Part model, mm, in its own coordinate system. Give positions to 0.01 mm unless a question says otherwise; leave off trailing zeros. Loops run counter-clockwise (first coordinate to the right, second up) from the corner with the lowest first, then second, coordinate; pieces in that order, holes last. Notation, with made-up numbers: M 45,60 L 88,60 A19 cw 88,88 Z; hole C 2,71 d2. An arc over 180 degrees is marked long. Put each result on its own line as item: value. Start each with the question number.
```python
from build123d import *

# Parameters (mm, degrees)
SKETCH1_R                        = 101.6
SKETCH1_R_2                      = 22.225
BOSS_EXTRUDE1_DEPTH              = 12.7
F_1_4_20_TAPPED_HOLE1_AT_2_COUNT = 2
F_1_4_20_TAPPED_HOLE1_AT_2_PITCH = 91.581002397
F_1_4_20_TAPPED_HOLE1_AT_3_COUNT = 2
F_1_4_20_TAPPED_HOLE1_AT_3_PITCH = 71.842048969
F_1_4_20_TAPPED_HOLE1_AT_4_COUNT = 2
F_1_4_20_TAPPED_HOLE1_AT_4_PITCH = 127
F_1_4_20_TAPPED_HOLE1_AT_5_COUNT = 2
F_1_4_20_TAPPED_HOLE1_AT_5_PITCH = 101.6
F_1_4_20_TAPPED_HOLE1_AT_6_COUNT = 2
F_1_4_20_TAPPED_HOLE1_AT_6_PITCH = 91.581002397
F_1_4_20_TAPPED_HOLE1_AT_7_COUNT = 2
F_1_4_20_TAPPED_HOLE1_AT_7_PITCH = 71.842048969
F_1_4_20_TAPPED_HOLE1_AT_8_COUNT = 2
F_1_4_20_TAPPED_HOLE1_AT_8_PITCH = 25.4


with BuildPart() as part:
    # Sketch1 → Boss-Extrude1 (new body)
    with BuildSketch(Plane.XY):
        Circle(SKETCH1_R)
        Circle(SKETCH1_R_2, mode=Mode.SUBTRACT)
    extrude(amount=BOSS_EXTRUDE1_DEPTH)

    # Sketch3 → 1/4-20 Tapped Hole1 (revolve, cut)
    with BuildSketch(Plane(origin=(-50.8, 0, 12.7), x_dir=(0, -1, 0), z_dir=(1, 0, 0))):
        Polygon((0, 0), (0, 12.7), (3.81, 12.7), (2.5527, 11.4427), (2.5527, 1.2573), (3.81, 0), align=None)
    f_1_4_20_tapped_hole1 = revolve(axis=Axis((-50.8, 0, 19.05), (0, 0, -1)), mode=Mode.SUBTRACT)

    # 1/4-20 Tapped Hole1 at 2: 1/4-20 Tapped Hole1 ×2
    with Locations(*[Vector(0.554700196, 0.832050294, 0) * (i * F_1_4_20_TAPPED_HOLE1_AT_2_PITCH) for i in range(1, F_1_4_20_TAPPED_HOLE1_AT_2_COUNT)]):
        add(f_1_4_20_tapped_hole1, mode=Mode.SUBTRACT)

    # 1/4-20 Tapped Hole1 at 3: 1/4-20 Tapped Hole1 ×2
    with Locations(*[Vector(0.707106781, 0.707106781, 0) * (i * F_1_4_20_TAPPED_HOLE1_AT_3_PITCH) for i in range(1, F_1_4_20_TAPPED_HOLE1_AT_3_COUNT)]):
        add(f_1_4_20_tapped_hole1, mode=Mode.SUBTRACT)

    # 1/4-20 Tapped Hole1 at 4: 1/4-20 Tapped Hole1 ×2
    with Locations(*[(i * F_1_4_20_TAPPED_HOLE1_AT_4_PITCH, 0, 0) for i in range(1, F_1_4_20_TAPPED_HOLE1_AT_4_COUNT)]):
        add(f_1_4_20_tapped_hole1, mode=Mode.SUBTRACT)

    # 1/4-20 Tapped Hole1 at 5: 1/4-20 Tapped Hole1 ×2
    with Locations(*[(i * F_1_4_20_TAPPED_HOLE1_AT_5_PITCH, 0, 0) for i in range(1, F_1_4_20_TAPPED_HOLE1_AT_5_COUNT)]):
        add(f_1_4_20_tapped_hole1, mode=Mode.SUBTRACT)

    # 1/4-20 Tapped Hole1 at 6: 1/4-20 Tapped Hole1 ×2
    with Locations(*[Vector(0.554700196, -0.832050294, 0) * (i * F_1_4_20_TAPPED_HOLE1_AT_6_PITCH) for i in range(1, F_1_4_20_TAPPED_HOLE1_AT_6_COUNT)]):
        add(f_1_4_20_tapped_hole1, mode=Mode.SUBTRACT)

    # 1/4-20 Tapped Hole1 at 7: 1/4-20 Tapped Hole1 ×2
    with Locations(*[Vector(0.707106781, -0.707106781, 0) * (i * F_1_4_20_TAPPED_HOLE1_AT_7_PITCH) for i in range(1, F_1_4_20_TAPPED_HOLE1_AT_7_COUNT)]):
        add(f_1_4_20_tapped_hole1, mode=Mode.SUBTRACT)

    # 1/4-20 Tapped Hole1 at 8: 1/4-20 Tapped Hole1 ×2
    with Locations(*[(-i * F_1_4_20_TAPPED_HOLE1_AT_8_PITCH, 0, 0) for i in range(1, F_1_4_20_TAPPED_HOLE1_AT_8_COUNT)]):
        add(f_1_4_20_tapped_hole1, mode=Mode.SUBTRACT)


solid = part.part
```
1) Mould opens along X. For faces 1 (the flat face through (-1, 24, 12.7)), 2 (the cylindrical face through (-53.33, 0.33, 6.42)), 3 (the cylindrical face through (-22.025, -99.184, 6.261)) say: +X half, -X half, draft (parallel to the pull), parting line (faces both ways), or undercut.
2) Band-saw the part on D-D on y = -19. Give the cut face in (x, z).
3) Wall check: L1, parallel to Y at x = 0, z = 7.75 (3 decimals); L2, parallel to X at y = 76.2, z = 6.75; L3, parallel to Y at x = -50.8, z = 6. Give the ranges that are in metal, low to high.
4) Band-saw the part on A-A on z = 5. State how many separate pieces and enclosed holes the cut face has, then the cut area to 3 significant figures.
5) Band-saw the part on B-B on x = -76.2. Give the cut face in (y, z), then the cut area to 3 significant figures.
6) Pin check, flat tips, straight feed: pin 1 Ø6.5 at (x, y) = (50.8, 0) entering from +Z; pin 2 Ø4 at (x, z) = (-54, 4.5) entering from +Y; pin 3 Ø6 at (x, y) = (0, 50.8) entering from -Z; pin 4 Ø4 at (x, y) = (-74.5, 44.5) entering from -Z. Stop position of each tip, or through.
Evaluation:
1. face 1: draft
1. face 2: undercut
1. face 3: parting line
2. outline: M -99.81,0 L -11.53,0 L -11.53,12.7 L -99.81,12.7 Z; M 11.53,0 L 99.81,0 L 99.81,12.7 L 11.53,12.7 Z
3. L1: -101.6 to -78.753, -73.647 to -53.353, -48.247 to -22.225, 22.225 to 48.247, 53.353 to 73.647, 78.753 to 101.6
3. L2: -67.2 to -2.55, 2.55 to 67.2
3. L3: -87.99 to -2.55, 2.55 to 87.99
4. separate pieces: 1
4. enclosed holes: 9
4. area: 30,700 mm2
5. outline: M -67.2,0 L -3.81,0 L -2.55,1.26 L -2.55,11.44 L -3.81,12.7 L -67.2,12.7 Z; M 2.55,1.26 L 3.81,0 L 67.2,0 L 67.2,12.7 L 3.81,12.7 L 2.55,11.44 Z
5. area: 1,640 mm2
6. pin 1: z = 12.14
6. pin 2: y = 87.28
6. pin 3: z = 0.81
6. pin 4: z = 0
